Geometry check sheet. Reference: the model listing, model coordinates, mm. Give positions to 0.01 mm unless a question says otherwise; leave off trailing zeros. Write each loop counter-clockwise with the first axis right and the second up, starting at its lowest first coordinate (ties: lowest second). Pieces come first, ordered by that corner, then holes. Notation, with made-up numbers: (-20, -14.75) -> (22, -14.75) arc R13 ccw to (22, 5.25) -> close; hole circle Ø1 at (-40, 0.25). An arc over 180 degrees is marked (long way). Write item = value, one per line. Start each with the question number.
1. Depth check by flat-ended pin: P1, Ø1.4, axis at x = 1.5, y = 2.5, coming from the -Z side; P2, Ø0.8, axis at x = 1.5, y = 4, coming from the +Z side; P3, Ø1, axis at y = -11.5, z = 15, coming from the +X side; P4, Ø1, axis at x = 1.5, z = 115.5, coming from the +Y side. Enter the tip coordinate at first touch or a pass-through.
2. Thickness scan on line 1 along Z through (x, y) = (1.45, -15); line 2 along Y through (x, z) = (2, 50); line 3 along Y through (x, z) = (1.65, 141). Record the ranges inside material, lowest first.
3. Cross-section at D-D, the plane z = 48. Record the cut outline in (x, y), plus the area to 3 significant figures.
4. Cross-section at A-A, the plane y = 3. Record the cut outline in (x, z), plus the area to 3 significant figures.
5. Cross-section at C-C, the plane y = -14. Record the cut outline in (x, z), plus the area to 3 significant figures.
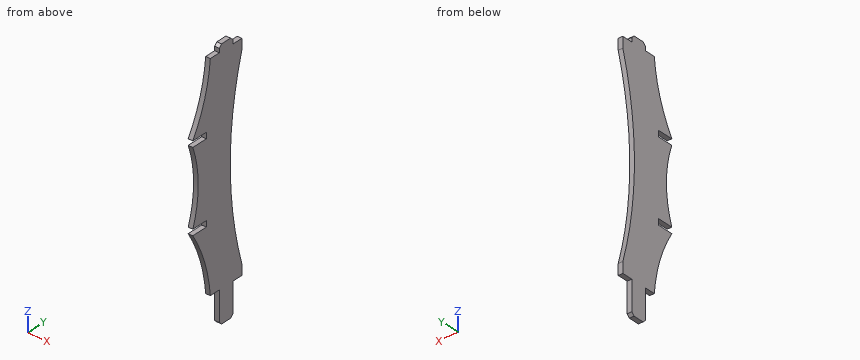
```python
from build123d import *

# Parameters (mm, degrees)
BOSS_EXTRUDE1_DEPTH = 2.75
CHAMFER1_SIZE       = 1.5875


with BuildPart() as part:
    # Sketch1 → Boss-Extrude1 (new body)
    with BuildSketch(Plane.YZ):
        with BuildLine():
            Line((-9.525, 19.05), (-15.875, 19.05))
            ThreePointArc((-15.875, 19.05), (-19.876556287, 38.808169282), (-28.241659516, 57.15))
            Line((-28.241659516, 57.15), (-18.716659516, 57.15))
            Line((-18.716659516, 57.15), (-18.716659516, 60.65))
            Line((-18.716659516, 60.65), (-28.241659516, 60.65))
            ThreePointArc((-28.241659516, 60.65), (-24.444713557, 82.55), (-28.241659516, 104.45))
            Line((-28.241659516, 104.45), (-18.716659516, 104.45))
            Line((-18.716659516, 104.45), (-18.716659516, 107.95))
            Line((-18.716659516, 107.95), (-28.241659516, 107.95))
            ThreePointArc((-28.241659516, 107.95), (-19.876556287, 126.291830718), (-15.875, 146.05))
            Line((-15.875, 146.05), (-9.525, 146.05))
            Line((-9.525, 146.05), (-9.525, 150.05))
            Line((-9.525, 150.05), (0, 150.05))
            Line((0, 150.05), (0, 146.05))
            Line((0, 146.05), (6.35, 146.05))
            Line((6.35, 146.05), (6.35, 139.7))
            ThreePointArc((6.35, 139.7), (-1.810573999, 82.55), (6.35, 25.4))
            Line((6.35, 25.4), (6.35, 19.05))
            Line((6.35, 19.05), (0, 19.05))
            Line((0, 19.05), (0, 0))
            Line((0, 0), (-9.525, 0))
            Line((-9.525, 0), (-9.525, 19.05))
        make_face()
    extrude(amount=BOSS_EXTRUDE1_DEPTH)

    # Chamfer1
    chamfer1_edges = [part.edges().sort_by_distance(p)[0] for p in [
        (1.375, 0, 0),
        (1.375, -9.525, 0),
        (1.375, -9.525, 150.05),
        (1.375, 0, 150.05),
    ]]
    chamfer(chamfer1_edges, length=CHAMFER1_SIZE)


solid = part.part
```
Answers:
q1.P1 = 19.05
q1.P2 = 146.05
q1.P3 = through
q1.P4 = 0.95
q2.line_1 = 19.05 to 146.05
q2.line_2 = -24.37 to 0.8
q2.line_3 = -16.46 to 6.35
q3.outline = (0, -23.44) -> (2.75, -23.44) -> (2.75, 1.13) -> (0, 1.13) -> close
q3.area = 67.6 mm^2
q4.outline = (0, 19.05) -> (2.75, 19.05) -> (2.75, 38.49) -> (0, 38.49) -> close; (0, 126.61) -> (2.75, 126.61) -> (2.75, 146.05) -> (0, 146.05) -> close
q4.area = 107 mm^2
q5.outline = (0, 19.05) -> (2.75, 19.05) -> (2.75, 146.05) -> (0, 146.05) -> close
q5.area = 349 mm^2
